```python
from build123d import *

# Parameters (mm, degrees)
BOSS_EXTRUDE1_DEPTH = 5
CUT_EXTRUDE1_REACH  = 114.056
CUT_EXTRUDE2_REACH  = 111.68
FILLET1_R           = 5.25
DRAFT1_ANGLE        = -1


with BuildPart() as part:
    # Sketch1 → Boss-Extrude1 (new body)
    with BuildSketch(Plane(origin=(0, 0, 0), x_dir=(1, 0, 0), z_dir=(0, 1, 0))):
        Polygon((0, 0), (7.835950564, 14.23), (111.035815461, 14.23), (103.199864898, 0), align=None)
    extrude(amount=BOSS_EXTRUDE1_DEPTH)

    # Sketch2 → Cut-Extrude1 (cut, up to next)
    with BuildSketch(Plane(origin=(0, 5, 0), x_dir=(1, 0, 0), z_dir=(0, 1, 0)), mode=Mode.PRIVATE) as cut_extrude1_sk1:
        Polygon((104.909775718, 3.105179235), (103.070238426, 4.118146436), (108.638473467, 14.23), (111.035815461, 14.23), align=None)
    cut_extrude1_tool1 = extrude(cut_extrude1_sk1.sketch, amount=-CUT_EXTRUDE1_REACH, mode=Mode.PRIVATE) & part.part
    add(cut_extrude1_tool1.solids().sort_by_distance((106.930417, 5, -8.916805))[0], mode=Mode.SUBTRACT)

    # Sketch4 → Cut-Extrude2 (cut, up to next)
    with BuildSketch(Plane(origin=(0, 5, 0), x_dir=(1, 0, 0), z_dir=(0, 1, 0)), mode=Mode.PRIVATE) as cut_extrude2_sk1:
        Polygon((108.638473467, 14.23), (107.2909351, 11.782885153), (102.847001464, 14.23), align=None)
    cut_extrude2_tool1 = extrude(cut_extrude2_sk1.sketch, amount=-CUT_EXTRUDE2_REACH, mode=Mode.PRIVATE) & part.part
    add(cut_extrude2_tool1.solids().sort_by_distance((106.258803, 5, -13.414295))[0], mode=Mode.SUBTRACT)

    # Fillet1
    fillet1_edges = [part.edges().sort_by_distance(p)[0] for p in [
        (103.199864898, 2.5, 0),
    ]]
    fillet(fillet1_edges, radius=FILLET1_R)

    # Draft1
    draft1_faces = [part.faces().sort_by_distance(p)[0] for p in [
        (50.048748296, 2.5, 0),
        (104.80305777, 2.5, -2.911380615),
        (102.76838647, 2.5, -0.730171766),
    ]]
    draft(draft1_faces, Plane.ZX.offset(5), DRAFT1_ANGLE)


solid = part.part
```
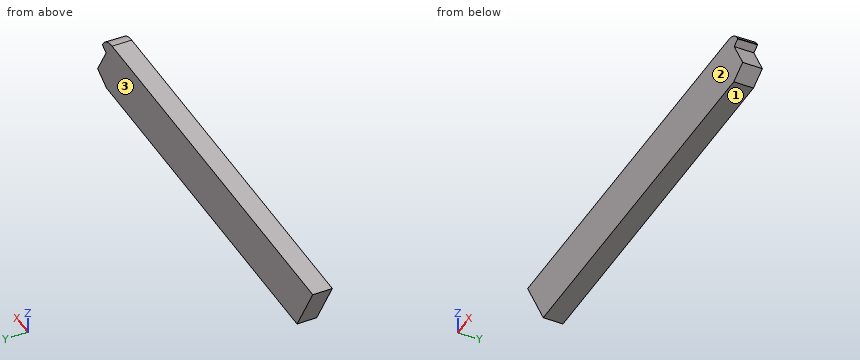
Here's how the part is built. I have some questions about the finished solid (model axes, mm). Face numbers are marked on the shaded views. Give positions to 0.01 mm unless a question says otherwise; leave off trailing zeros. Loops run counter-clockwise (first coordinate to the right, second up) from the corner with the lowest first, then second, coordinate; pieces in that order, holes last. Notation, with made-up numbers: M 27.5,-12 L 46.5,-12 A20 cw 46.5,-2 Z; hole C -3,58.25 d7. An arc over 180 degrees is marked long. Put each result on its own line as item: value. Start each with the question number.
(1) I need wall thicknesses on line 1 along Z through (x, y) = (44.5, 0.75); line 2 along X through (y, z) = (1.1, -3); line 3 along X through (y, z) = (3.9, -6). Which ranges of each line are inside material? Lowest first, please. Write a range as [from, to].
(2) Will these pins go through, and if not, where does the flat tip stop? pin 1 Ø1.5 at (x, y) = (62.5, 4) entering from +Z; pin 2 Ø3 at (y, z) = (1.5, -4.5) entering from +X.
(3) I want a section at A-A on y = 1.9. Please give me the cut outline in (x, z), then the cut area to 3 significant figures.
(4) I want a section at B-B on z = -12.75. Please give me the cut outline in (x, y), then the cut area to 3 significant figures.
(5) I want a section at C-C on z = -7. Please give me the cut outline in (x, y), then the cut area to 3 significant figures.
(6) If we mould it in two halves opening along Y, with no side actions, what happens to the marked faces 1, 2 and 3? For each: +Y half, -Y half, draft (parallel to the pull), parting line (faces both ways), or undercut.
Answer block:
1. line 1: [-14.23, -0.07]
1. line 2: [1.65, 104.77]
1. line 3: [3.3, 104.11]
2. pin 1: z = 0
2. pin 2: x = 104.87
3. outline: M 0.03,-0.05 L 7.84,-14.23 L 102.85,-14.23 L 107.29,-11.78 L 103.07,-4.12 L 104.86,-3.13 L 104.65,-2.74 A5.2 ccw 100.1,-0.05 Z
3. area: 1,430 mm^2
4. outline: M 7.02,0 L 105.53,0 L 105.53,5 L 7.02,5 Z
4. area: 493 mm^2
5. outline: M 3.85,0 L 104.66,0 L 104.66,5 L 3.85,5 Z
5. area: 504 mm^2
6. face 1: draft
6. face 2: -Y half
6. face 3: +Y half
